```python
from build123d import *

# Parameters (mm, degrees)
SKETCH1_R                       = 5.334
BOSS_EXTRUDE1_DEPTH             = 19.05
F_3_16_0_1875_DOWEL_HOLE2_D     = 4.7625
F_3_16_0_1875_DOWEL_HOLE2_DEPTH = 9.525
F_3_16_0_1875_DOWEL_HOLE2_TIP   = 1.430799349
F_5_0MM_DOWEL_HOLE2_D           = 5
F_5_0MM_DOWEL_HOLE2_DEPTH       = 9.525
F_5_0MM_DOWEL_HOLE2_TIP         = 1.502151548
F_10_32_TAPPED_HOLE1_REACH      = 26.836
F_10_32_TAPPED_HOLE1_BORE_R     = 2.0193


with BuildPart() as part:
    # Sketch1 → Boss-Extrude1 (new body)
    with BuildSketch(Plane(origin=(0, 0, 0), x_dir=(1, 0, 0), z_dir=(0, 1, 0))):
        with Locations(Location((0, 0, 0), (0, 0, 90))):
            Circle(SKETCH1_R)
    extrude(amount=BOSS_EXTRUDE1_DEPTH)

    # 3/16 (0.1875) Dowel Hole2
    with Locations(Plane(origin=(0, 19.05, 0), x_dir=(1, 0, 0), z_dir=(0, 1, 0))):
        with Locations((0, 0)):
            Hole(F_3_16_0_1875_DOWEL_HOLE2_D / 2, depth=F_3_16_0_1875_DOWEL_HOLE2_DEPTH)
            with Locations((0, 0, -(F_3_16_0_1875_DOWEL_HOLE2_DEPTH + F_3_16_0_1875_DOWEL_HOLE2_TIP / 2))):  # 118° drill point
                Cone(0, F_3_16_0_1875_DOWEL_HOLE2_D / 2, F_3_16_0_1875_DOWEL_HOLE2_TIP, mode=Mode.SUBTRACT)

    # Ø5.0mm Dowel Hole2
    with Locations(Plane(origin=(0, 0, 0), x_dir=(-1, 0, 0), z_dir=(0, -1, 0))):
        with Locations((0, 0)):
            Hole(F_5_0MM_DOWEL_HOLE2_D / 2, depth=F_5_0MM_DOWEL_HOLE2_DEPTH)
            with Locations((0, 0, -(F_5_0MM_DOWEL_HOLE2_DEPTH + F_5_0MM_DOWEL_HOLE2_TIP / 2))):  # 118° drill point
                Cone(0, F_5_0MM_DOWEL_HOLE2_D / 2, F_5_0MM_DOWEL_HOLE2_TIP, mode=Mode.SUBTRACT)

    # #10-32 Tapped Hole1 bore → #10-32 Tapped Hole1 (cut, up to next)
    with BuildSketch(Plane.XY.offset(9.681668378), mode=Mode.PRIVATE) as f_10_32_tapped_hole1_sk1:
        with Locations((0, 15.621)):
            Circle(F_10_32_TAPPED_HOLE1_BORE_R)
    f_10_32_tapped_hole1_tool1 = extrude(f_10_32_tapped_hole1_sk1.sketch, amount=-F_10_32_TAPPED_HOLE1_REACH, mode=Mode.PRIVATE) & part.part
    # #10-32 Tapped Hole1 bore → #10-32 Tapped Hole1 (cut, up to next)
    with BuildSketch(Plane.XY.offset(9.681668378), mode=Mode.PRIVATE) as f_10_32_tapped_hole1_sk2:
        with Locations((0, 3.429)):
            Circle(F_10_32_TAPPED_HOLE1_BORE_R)
    f_10_32_tapped_hole1_tool2 = extrude(f_10_32_tapped_hole1_sk2.sketch, amount=-F_10_32_TAPPED_HOLE1_REACH, mode=Mode.PRIVATE) & part.part
    add(f_10_32_tapped_hole1_tool1.solids().sort_by_distance((0, 15.621, 9.681668))[0], mode=Mode.SUBTRACT)
    add(f_10_32_tapped_hole1_tool2.solids().sort_by_distance((0, 3.429, 9.681668))[0], mode=Mode.SUBTRACT)


solid = part.part
```
Input: part model. Units: mm. Frame: model coordinates. A direction names the side the tool comes from. Coordinates: 2 decimals unless noted, no trailing zeros. Loops run counter-clockwise (first coordinate to the right, second up) from the corner with the lowest first, then second, coordinate; pieces in that order, holes last. Notation, with made-up numbers: M -9.5,60 L -4.5,60 A14 ccw -4.5,67 Z; hole C 18.5,-39.75 d9. An arc over 180 degrees is marked long. Use a Markdown table: item, result. Add a question column.
1) Section C-C, the plane y = 12.25. Return the cut outline in (x, z), plus the area to 3 significant figures.
2) Draft query along Y for faces 4 (the flat face through (-2.45, 0, -1.11)), 5 (the flat face through (1.1, 19.05, -2.3)), 6 (the cylindrical face through (1.926, 16.228, 3.328)). Return one class per face: +Y half, -Y half, draft (parallel to the pull), parting line (faces both ways), or undercut.
3) Set-up query: faces 1 (the cylindrical face through (1.926, 4.036, 3.432)), 2 (the cylindrical face through (-0.33, 4.83, -2.48)), 3 (the cylindrical face through (2.04, 9.39, -4.93)). Return all of +Z, -Z, +X, -X, +Y, -Y with unobstructed straight access to the full face (end or side cutting, diameter ignored); none if empty.
4) Pin query (flat end, axial travel): P1, Ø1, axis at x = -3.5, z = -1.5, coming from the -Y side; P2, Ø4, axis at y = 5.5, z = -3.5, coming from the +X side; P3, Ø4, axis at x = 3, y = 16, coming from the -Z side; P4, Ø2, axis at y = 10, z = -3, coming from the -X side. Return the tip coordinate at first contact, or that it passes through.
5) Section A-A, the plane z = 0. Return the cut outline in (x, y) (3 decimals).
6) Section D-D, the plane z = 3.25. Return the cut outline in (x, y), plus the area to 3 significant figures.
7) Section B-B, the plane x = 0. Return the cut outline in (y, z) (3 decimals).
8) Line query: L1, parallel to Y at x = 0, z = 4.3; L2, parallel to X at y = 18.25, z = 0.25; L3, parallel to X at y = 9.25, z = 2. Output: solid intervals per line, ascending. Write a range as from..to.
Answer below:
| question | item | result |
|---|---|---|
| 1 | outline | C 0,0 d10.67; hole C 0,0 d4.76 |
| 1 | area | 71.6 mm2 |
| 2 | face 4 | -Y half |
| 2 | face 5 | +Y half |
| 2 | face 6 | undercut |
| 3 | face 1 | +Z |
| 3 | face 2 | -Y |
| 3 | face 3 | +Y, -Y |
| 4 | P1 | y = 0 |
| 4 | P2 | x = 5.12 |
| 4 | P3 | z = -5.24 |
| 4 | P4 | x = -4.94 |
| 5 | outline | M -5.334,0 L -2.5,0 L -2.5,9.525 L -2.381,9.596 L -2.381,19.05 L -5.334,19.05 Z; M 2.381,9.596 L 2.5,9.525 L 2.5,0 L 5.334,0 L 5.334,19.05 L 2.381,19.05 Z |
| 6 | outline | M -4.23,0 L 4.23,0 L 4.23,19.05 L -4.23,19.05 Z; hole C 0,3.43 d4.04; hole C 0,15.62 d4.04 |
| 6 | area | 136 mm2 |
| 7 | outline | M 0,-5.334 L 19.05,-5.334 L 19.05,-2.381 L 9.596,-2.381 L 9.525,-2.5 L 0,-2.5 Z; M 0,2.5 L 1.41,2.5 L 1.41,5.334 L 0,5.334 Z; M 5.448,2.5 L 9.525,2.5 L 9.596,2.381 L 13.602,2.381 L 13.602,5.334 L 5.448,5.334 Z; M 17.64,2.381 L 19.05,2.381 L 19.05,5.334 L 17.64,5.334 Z |
| 8 | L1 | 0..1.41, 5.45..13.6, 17.64..19.05 |
| 8 | L2 | -5.33..-2.37, 2.37..5.33 |
| 8 | L3 | -4.94..-1.5, 1.5..4.94 |
